Answer from the drawing. Dimensions are ordinates in mm from the lowest x, y and z of the part. A direction names the side the tool comes from. Give positions to 0.01 mm unless a question says otherwise; leave off trailing zeros. Loops run counter-clockwise (first coordinate to the right, second up) from the corner with the lowest first, then second, coordinate; pieces in that order, holes last. Notation, with made-up numbers: (-34.75, 41) - (-6.75, 41) arc R12 cw to (-6.75, 62) - close; hole circle Ø4 at (84, 69.5). An arc over 180 degrees is marked (long way). Put each result on its own line as item: value. Start each with the question number.
1. For the marked faces 1, 2 and 3, determine the directions among +Z, -Z, +X, -X, +Y, -Y from which every point of the face is accessible in a straight line to the end or side of a thin tool.
2. A cutting plane is placed at C-C, the plane x = 4. Determine the outline of the cut face in (y, z).
3. Consider L1, parallel to X at y = 1.1, z = 4; L2, parallel to X at y = 5.45, z = 4; L3, parallel to Y at x = 2, z = 3.5. Determine where each line is inside the solid, lowest interval first. Write a range as from..to.
4. A cutting plane is placed at B-B, the plane z = 4. Determine the outline of the cut face in (x, y), plus the area to 3 significant figures.
5. Given pin 1 Ø1.5 at (y, z) = (5, 3) entering from +X; pin 2 Ø1.3 at (x, z) = (3.5, 4) entering from -Y; pin 3 Ø1 at (x, y) = (1.5, 1.5) entering from +Z; pin 4 Ø2 at (x, z) = (3, 3) entering from +Y, each flat-ended and moving along its own axis, determine where each tip first touches the part or whether it passes through.
6. For a pull along X with two mould halves and no side action, classify the marked faces 4, 5 and 6 as released by +X, released by -X, zero draft, split by the parting line, or undercut.
7. A cutting plane is placed at A-A, the plane y = 5.5. Determine the outline of the cut face in (x, z), plus the area to 3 significant figures.
8. A cutting plane is placed at D-D, the plane y = 4.7. Determine the outline of the cut face in (x, z), plus the area to 3 significant figures.
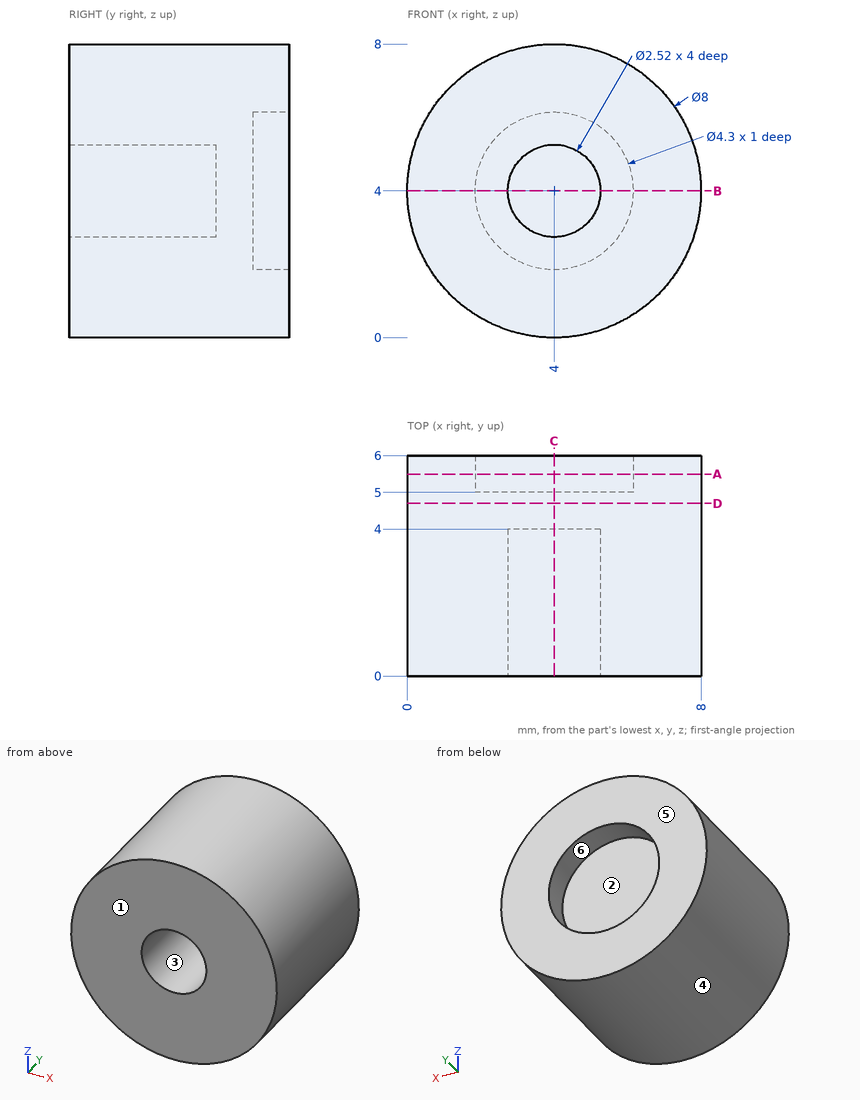
Return value:
1. face 1: +Z, -Z, +X, -X, -Y
1. face 2: +Y
1. face 3: -Y
2. outline: (0, 0) - (6, 0) - (6, 1.85) - (5, 1.85) - (5, 6.15) - (6, 6.15) - (6, 8) - (0, 8) - (0, 5.26) - (4, 5.26) - (4, 2.74) - (0, 2.74) - close
3. L1: x = 0..2.74, 5.26..8
3. L2: x = 0..1.85, 6.15..8
3. L3: y = 0..5
4. outline: (0, 0) - (2.74, 0) - (2.74, 4) - (5.26, 4) - (5.26, 0) - (8, 0) - (8, 6) - (6.15, 6) - (6.15, 5) - (1.85, 5) - (1.85, 6) - (0, 6) - close
4. area: 33.6 mm2
5. pin 1: stops at x = 7.99
5. pin 2: stops at y = 4
5. pin 3: stops at z = 7.46
5. pin 4: stops at y = 6
6. face 4: split by the parting line
6. face 5: zero draft
6. face 6: undercut
7. outline: circle Ø8 at (4, 4); hole circle Ø4.3 at (4, 4)
7. area: 35.7 mm2
8. outline: circle Ø8 at (4, 4)
8. area: 50.3 mm2
